from build123d import *

# Parameters (mm, degrees)
EXTRUDE_1_DEPTH     = 7
SKETCH_3_R          = 3.56
CUT_EXTRUDE_1_DEPTH = 20
SKETCH_4_R          = 1.35
CUT_EXTRUDE_2_DEPTH = 14
FILLET_1_R          = 5


with BuildPart() as part:
    # 草图1 → 凸台-拉伸1 (new, symmetric)
    with BuildSketch(Plane.XY):
        Polygon((-7.5, -18), (7.5, -18), (7.5, 23), (7.5, 26), (-2.5, 26), (-2.5, 44), (-7.5, 44), (-7.5, 26), (-7.5, 21), align=None)
    extrude(amount=EXTRUDE_1_DEPTH, both=True)

    # 草图3 → 切除-拉伸1 (cut)
    with BuildSketch(Plane(origin=(7.5, 0, 0), x_dir=(0, 0, -1), z_dir=(1, 0, 0))):
        with Locations((0, -10)):
            Circle(SKETCH_3_R)
        with Locations((0, 10)):
            Circle(SKETCH_3_R)
    extrude(amount=-CUT_EXTRUDE_1_DEPTH, mode=Mode.SUBTRACT)

    # 草图4 → 切除-拉伸2 (cut)
    with BuildSketch(Plane.XY.offset(7)):
        Circle(SKETCH_4_R)
    extrude(amount=-CUT_EXTRUDE_2_DEPTH, mode=Mode.SUBTRACT)

    # 圆角1
    fillet_1_edges = [part.edges().sort_by_distance(p)[0] for p in [
        (-5, 44, 7),
        (-5, 44, -7),
    ]]
    fillet(fillet_1_edges, radius=FILLET_1_R)


solid = part.part
The listing builds one solid part. Answer for the finished solid, in the listing's coordinates (mm). A direction names the side the tool comes from. Coordinates: 2 decimals unless noted, no trailing zeros. Order: outer loops, then holes, each group sorted by start corner. A loop starts at its lowest first (then second) coordinate and runs counter-clockwise, first axis right, second up.
Q1. A cutting plane is placed at A-A, the plane z = 0. Write down the section's boundary in (x, y), and give its area (3 significant figures).
Q2. Given P1, Ø2, axis at x = 4.5, z = 5, coming from the +Y side; P2, Ø2, axis at y = 35.5, z = 2.5, coming from the +X side, each flat-ended and moving along its own axis, determine where each tip first touches the part or whether it passes through.
Q3. A cutting plane is placed at D-D, the plane x = 2.5. Write down the section's boundary in (y, z), and give its area (3 significant figures).
Q4. Which of the six approach directions +Z, -Z, +X, -X, +Y, -Y give full straight-line access (tool end or side, diameter ignored) to faces 1 (the face through (-2.5, 35, 0)), 2 (the face through (0, 5, -7))?
Q5. For a pull along Y with two mould halves and no side action, classify faces 3 (the face through (0, -18, 0)), 4 (the face through (0.105, 6.525, 0.772)), 5 (the face through (-5, 42, 6)), 6 (the face through (0, 5, 7)) as pulls with the +Y half, pulls with the -Y half, needs draft (parallel to the pull), parting line crosses it, or undercut.
Q6. A cutting plane is placed at C-C, the plane y = -10. Write down the section's boundary in (x, z).
Q7. Consider line 1 (Y direction, x = -1, z = 3); line 2 (Y direction, x = 0, z = -3); line 3 (Y direction, x = -2, z = 4). Determine where each line is inside the solid, lowest interval first.
Q8. A cutting plane is placed at B-B, the plane x = 0. Write down the section's boundary in (y, z).
Answers follow:
1. outline: (-7.5, -18) - (7.5, -18) - (7.5, -13.56) - (-7.5, -13.56) - close; (-7.5, -6.44) - (7.5, -6.44) - (7.5, 6.44) - (-7.5, 6.44) - close; (-7.5, 13.56) - (7.5, 13.56) - (7.5, 26) - (-2.5, 26) - (-2.5, 44) - (-7.5, 44) - close; hole circle Ø2.7 at (0, 0)
1. area: 531 mm2
2. P1: stops at y = 26
2. P2: stops at x = -2.5
3. outline: (-18, -7) - (26, -7) - (26, 7) - (-18, 7) - close; hole circle Ø7.12 at (-10, 0); hole circle Ø7.12 at (10, 0)
3. area: 536 mm2
4. face 1: +Z, -Z, +X, +Y
4. face 2: -Z, +X, -X, +Y, -Y
5. face 3: pulls with the -Y half
5. face 4: undercut
5. face 5: pulls with the +Y half
5. face 6: needs draft
6. outline: (-7.5, -7) - (7.5, -7) - (7.5, -3.56) - (-7.5, -3.56) - close; (-7.5, 3.56) - (7.5, 3.56) - (7.5, 7) - (-7.5, 7) - close
7. line 1: y = -18 to -11.92, -8.08 to -0.91, 0.91 to 8.08, 11.92 to 26
7. line 2: y = -18 to -11.92, -8.08 to -1.35, 1.35 to 8.08, 11.92 to 26
7. line 3: y = -18 to 26
8. outline: (-18, -7) - (-1.35, -7) - (-1.35, 7) - (-18, 7) - close; (1.35, -7) - (26, -7) - (26, 7) - (1.35, 7) - close; hole circle Ø7.12 at (-10, 0); hole circle Ø7.12 at (10, 0)
